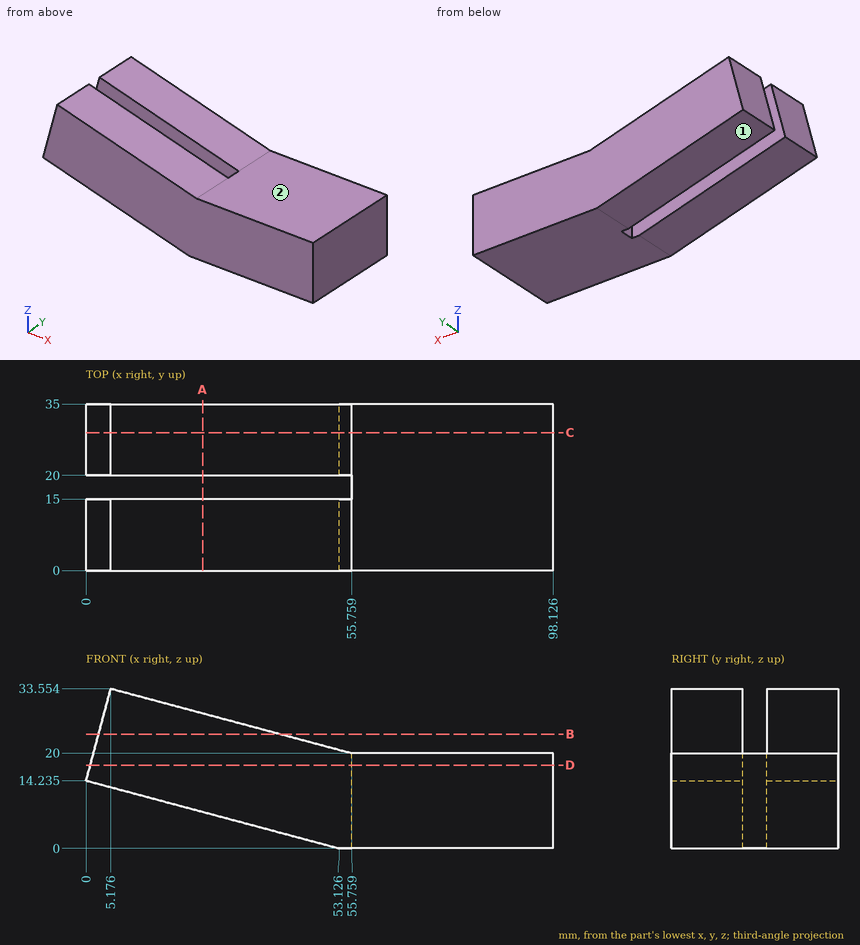
Check sheet for the drawn part. Datum: minimum x, y, z corner. Units: mm. A direction names the side the tool comes from. Coordinates: 2 decimals unless noted, no trailing zeros. Write each loop counter-clockwise with the first axis right and the second up, starting at its lowest first coordinate (ties: lowest second). Pieces come first, ordered by that corner, then holes. Notation, with made-up numbers: (-6.75, -1.75) - (46.25, -1.75) arc R15 cw to (46.25, 13.25) - close; hole circle Ø8 at (53.5, 24). An arc over 180 degrees is marked (long way). Answer as a JSON object with one key per item and string values.
(1) Tool access check on the marked faces 1 and 2. Record the directions out of +Z, -Z, +X, -X, +Y, -Y that give a thin tool (end or side, any length) a straight path to the whole face; none if there is none.
Report:
{"face 1": "-Z, -X, +Y, -Y", "face 2": "+Z, +X, +Y, -Y"}
(2) Cross-section at B-B on z = 24. Record the cut outline in (x, y), plus the area to 3 significant figures.
Report:
{"outline": "(2.62, 0) - (40.83, 0) - (40.83, 15) - (2.62, 15) - close; (2.62, 20) - (40.83, 20) - (40.83, 35) - (2.62, 35) - close", "area": "1,150 mm^2"}
(3) Gauge pin test, flat ends, axial feed: pin 1 Ø17.5 at (x, y) = (82, 22.5) entering from +Z; pin 2 Ø3 at (x, z) = (30.5, 26) entering from -Y; pin 3 Ø4 at (x, y) = (56.5, 18.5) entering from +Z (1 decimal); pin 4 Ø5 at (x, y) = (31, 18.5) entering from +Z. Record the tip position at first contact, or that the pin passes through.
Report:
{"pin 1": "z = 20", "pin 2": "y = 0", "pin 3": "z = 20.2", "pin 4": "z = 27.17"}
(4) Cross-section at D-D on z = 17.5. Record the cut outline in (x, y) (1 decimal).
Report:
{"outline": "(0.9, 0) - (98.1, 0) - (98.1, 35) - (0.9, 35) - (0.9, 20) - (55.8, 20) - (55.8, 15) - (0.9, 15) - close"}
(5) Thickness scan on line 1 along Y through (x, z) = (18.5, 16); line 2 along Z through (x, y) = (59.5, 20); line 3 along Z through (x, y) = (30, 2.5). Record the ranges inside material, lowest first.
Report:
{"line 1": "0 to 15, 20 to 35", "line 2": "0 to 20", "line 3": "6.2 to 26.9"}
(6) Cross-section at C-C on y = 29. Record the cut outline in (x, z) (1 decimal).
Report:
{"outline": "(0, 14.2) - (53.1, 0) - (98.1, 0) - (98.1, 20) - (55.8, 20) - (5.2, 33.6) - close"}
(7) Cross-section at A-A on x = 24.5. Record the cut outline in (y, z).
Report:
{"outline": "(0, 7.67) - (15, 7.67) - (15, 28.38) - (0, 28.38) - close; (20, 7.67) - (35, 7.67) - (35, 28.38) - (20, 28.38) - close"}
